Design review of the part built by this model. Coordinates are the model's own, in mm. A direction names the side the tool comes from. Round coordinates to 2 decimals unless told otherwise and drop trailing zeros. Order: outer loops, then holes, each group sorted by start corner. A loop starts at its lowest first (then second) coordinate and runs counter-clockwise, first axis right, second up. Notation, with made-up numbers: (12.5, -20.75) - (33.5, -20.75) arc R21 ccw to (33.5, -7.75) - close; hole circle Ø6 at (-39.5, -30.75). An arc over 180 degrees is marked (long way). Answer as a JSON object with one key per item and string values. Group by question number.
from build123d import *

# Parameters (mm, degrees)
BASE_FLANGIA1_DEPTH            = 3.175
BORDO_FLANGIA1_STRIP_W         = 14.1732
BORDO_FLANGIA1_STRIP_H         = 3.175
BORDO_FLANGIA1_STRIP_CUT_DEPTH = 42.0624
BORDO_FLANGIA1_DEPTH           = 42.0624
RIPETIZIONE_A_L1_COUNT         = 3
RIPETIZIONE_A_L1_PITCH         = 19.05
RIPETIZIONE_A_L1_COUNT_DIR2    = 3
RIPETIZIONE_A_L1_PITCH_DIR2    = 12.7
RIPETIZIONECIRCOLARE1_COUNT    = 6
SCHIZZO13_R                    = 6.096
TAGLIO_ESTRUSIONE1_DEPTH       = 10


# Sheet-metal steps are written as plain solids
with BuildPart() as part:
    # Schizzo1 → Base-Flangia1 (new body)
    with BuildSketch(Plane.XY):
        with BuildLine():
            Line((-21.0312, 0), (21.0312, 0))
            Line((21.0312, 0), (21.0312, 31.1912))
            ThreePointArc((21.0312, 31.1912), (0, 52.2224), (-21.0312, 31.1912))
            Line((-21.0312, 31.1912), (-21.0312, 0))
        make_face()
    extrude(amount=-BASE_FLANGIA1_DEPTH)

    # Bordo-Flangia1 strip (across the edge) → Bordo-Flangia1 strip cut (cut)
    with BuildSketch(Plane.YZ.offset(-21.0312)):
        with Locations((-3.175, -1.5875)):
            Rectangle(BORDO_FLANGIA1_STRIP_W, BORDO_FLANGIA1_STRIP_H)
    extrude(amount=BORDO_FLANGIA1_STRIP_CUT_DEPTH, mode=Mode.SUBTRACT)

    # Bordo-Flangia1 section (across the edge) → Bordo-Flangia1 (add)
    with BuildSketch(Plane.YZ.offset(-21.0312)):
        with BuildLine():
            Line((0, 0.7366), (0, 51.435))
            Line((0, 51.435), (3.175, 51.435))
            Line((3.175, 51.435), (3.175, 0.7366))
            ThreePointArc((3.175, 0.7366), (3.390745145, 0.215745145), (3.9116, 0))
            Line((3.9116, 0), (3.9116, -3.175))
            ThreePointArc((3.9116, -3.175), (1.145681115, -2.029318885), (0, 0.7366))
        make_face()
    extrude(amount=BORDO_FLANGIA1_DEPTH)

    # Schizzo9 → Foro filettato M3x0.5-1 (revolve, cut)
    with BuildSketch(Plane(origin=(-12.7, 3.175, 6.35), x_dir=(0, 0, 1), z_dir=(1, 0, 0))):
        Polygon((0, 0), (0, 8.251075774), (1.25, 7.5), (1.25, 0), align=None)
    foro_filettato_m3x0_5_1 = revolve(axis=Axis((-12.7, 9.525, 6.35), (0, -1, 0)), mode=Mode.SUBTRACT)

    # Ripetizione a L1: Foro filettato M3x0.5-1 3 × 3
    with Locations(*[(j * RIPETIZIONE_A_L1_PITCH_DIR2, 0, i * RIPETIZIONE_A_L1_PITCH) for i in range(RIPETIZIONE_A_L1_COUNT) for j in range(RIPETIZIONE_A_L1_COUNT_DIR2) if (i, j) != (0, 0)]):
        add(foro_filettato_m3x0_5_1, mode=Mode.SUBTRACT)

    # Schizzo11 → Foro filettato M3x0.5-2 (revolve, cut)
    with BuildSketch(Plane(origin=(-17.3812, 31.1912, -3.175), x_dir=(0, 1, 0), z_dir=(1, 0, 0))):
        Polygon((0, 0), (0, 8.251075774), (1.25, 7.5), (1.25, 0), align=None)
    foro_filettato_m3x0_5_2 = revolve(axis=Axis((-17.3812, 31.1912, -9.525), (0, 0, 1)), mode=Mode.SUBTRACT)

    # RipetizioneCircolare1: Foro filettato M3x0.5-2 ×6 about axis, 2 skipped
    ripetizionecircolare1_axis = Axis((0, 31.1912, 0), (0, 0, 1))
    add([foro_filettato_m3x0_5_2.rotate(ripetizionecircolare1_axis, i * 360 / RIPETIZIONECIRCOLARE1_COUNT) for i in range(1, RIPETIZIONECIRCOLARE1_COUNT) if i not in (2, 4)], mode=Mode.SUBTRACT)

    # Schizzo13 → Taglio-Estrusione1 (cut)
    with BuildSketch(Plane(origin=(0, 0, -3.175), x_dir=(-1, 0, 0), z_dir=(0, 0, -1))):
        with Locations((0, 38.227)):
            Circle(SCHIZZO13_R)
    extrude(amount=-TAGLIO_ESTRUSIONE1_DEPTH, mode=Mode.SUBTRACT)


solid = part.part
1. Take a section at D-D, the plane y = 7. Give the boundary of the cut face in (x, z) (3 decimals).
2. Take a section at C-C, the plane x = -9. Give the boundary of the cut face in (y, z) (3 decimals).
3. Take a section at A-A, the plane z = 44.45. Give the boundary of the cut face in (x, y) (3 decimals), then the cut area to 3 significant figures.
4. Clearance check with flat-ended pins moving along their axes: P1, Ø2, axis at x = 0, z = 44.45, coming from the +Y side; P2, Ø1.5, axis at x = 15, y = 15, coming from the +Z side; P3, Ø3, axis at x = 12.7, z = 44.45, coming from the +Y side (3 decimals). State where each tip first meets the part, or that it passes through.
5. Take a section at B-B, the plane x = 0. Give the boundary of the cut face in (y, z) (3 decimals), then the cut area to 3 significant figures.
6. To check wall thickness, follow line 1 (X direction, y = 0.9, z = 25.4); line 2 (Z direction, x = 12.7, y = 0.85) (3 decimals); line 3 (Z direction, x = 0, y = 1.4) (3 decimals). State the ranges of each line that lie inside material, in increasing order. Write a range as from..to.
7. Mouldability with a two-part tool opening along Y and no side actions: class faces 3 (the cylindrical face through (17.44, 32.44, -1.61)), 4 (the cylindrical face through (0.462, 52.217, -1.565)), 5 (the cylindrical face through (-0.294, 1.176, -2.06)), 6 (the cylindrical face through (12.65, 1.61, 43.2)) as pulls with the +Y half, pulls with the -Y half, needs draft (parallel to the pull), parting line crosses it, or undercut.
8. Tool access review of faces 1 (the flat face through (0, 28, 0)), 2 (the flat face through (0, 28, -3.175)): name each direction out of +Z, -Z, +X, -X, +Y, -Y from which nothing blocks a thin tool from reaching the whole face with its end or side.
Response values:
{
 "1": {"outline": "(-21.031, -3.175) - (21.031, -3.175) - (21.031, 0) - (-21.031, 0) - close"},
 "2": {"outline": "(0, 0.737) arc R3.912 ccw to (3.912, -3.175) - (14.928, -3.175) - (14.928, 0) - (3.912, 0) arc R0.737 cw to (3.175, 0.737) - (3.175, 51.435) - (0, 51.435) - close; (17.35, -3.175) - (45.033, -3.175) - (45.033, 0) - (17.35, 0) - close; (47.455, -3.175) - (50.199, -3.175) - (50.199, 0) - (47.455, 0) - close"},
 "3": {"outline": "(-21.031, 0) - (-13.95, 0) - (-13.95, 3.175) - (-21.031, 3.175) - close; (-11.45, 0) - (-1.25, 0) - (-1.25, 3.175) - (-11.45, 3.175) - close; (1.25, 0) - (11.45, 0) - (11.45, 3.175) - (1.25, 3.175) - close; (13.95, 0) - (21.031, 0) - (21.031, 3.175) - (13.95, 3.175) - close", "area": "110 mm2"},
 "4": {"P1": "through", "P2": "z = 0", "P3": "y = 3.175"},
 "5": {"outline": "(0, 0.737) arc R3.912 ccw to (3.912, -3.175) - (32.131, -3.175) - (32.131, 0) - (3.912, 0) arc R0.737 cw to (3.175, 0.737) - (3.175, 5.1) - (0, 5.1) - close; (0, 7.6) - (3.175, 7.6) - (3.175, 24.15) - (0, 24.15) - close; (0, 26.65) - (3.175, 26.65) - (3.175, 43.2) - (0, 43.2) - close; (0, 45.7) - (3.175, 45.7) - (3.175, 51.435) - (0, 51.435) - close; (44.323, -3.175) - (52.222, -3.175) - (52.222, 0) - (44.323, 0) - close", "area": "263 mm2"},
 "6": {"line 1": "-21.03..-13.95, -11.45..-1.25, 1.25..11.45, 13.95..21.03", "line 2": "-1.698..5.1, 7.6..24.15, 26.65..43.2, 45.7..51.435", "line 3": "-2.262..5.1, 7.6..24.15, 26.65..43.2, 45.7..51.435"},
 "7": {"face 3": "undercut", "face 4": "pulls with the +Y half", "face 5": "pulls with the -Y half", "face 6": "needs draft"},
 "8": {"face 1": "+Z, +X, -X, +Y", "face 2": "-Z, +X, -X, +Y, -Y"}
}
